from build123d import *

# Parameters (mm, degrees)
ESQUISSE1_W             = 160
ESQUISSE1_H             = 80
BOSS_EXTRU_1_DEPTH      = 2
ENL_V_MAT_EXTRU_2_DEPTH = 2
ENL_V_MAT_EXTRU_3_DEPTH = 2
ENL_V_MAT_EXTRU_4_REACH = 4
ESQUISSE8_W             = 8
ESQUISSE8_H             = 48


with BuildPart() as part:
    # Esquisse1 → Boss.-Extru.1 (new body)
    with BuildSketch(Plane(origin=(0, 0, 0), x_dir=(1, 0, 0), z_dir=(0, 1, 0))):
        with Locations((80, 40)):
            Rectangle(ESQUISSE1_W, ESQUISSE1_H)
    extrude(amount=BOSS_EXTRU_1_DEPTH)

    # Esquisse2 → Enlèv. mat.-Extru.2 (cut)
    with BuildSketch(Plane(origin=(0, 2, 0), x_dir=(1, 0, 0), z_dir=(0, 1, 0))):
        Polygon((0, 50), (30, 80), (0, 80), align=None)
        Polygon((130, 80), (160, 50), (160, 80), align=None)
        Polygon((130, 0), (160, 30), (160, 0), align=None)
        Polygon((0, 30), (30, 0), (0, 0), align=None)
    extrude(amount=-ENL_V_MAT_EXTRU_2_DEPTH, mode=Mode.SUBTRACT)

    # Esquisse7 → Enlèv. mat.-Extru.3 (cut)
    with BuildSketch(Plane(origin=(0, 2, 0), x_dir=(1, 0, 0), z_dir=(0, 1, 0))):
        with BuildLine():
            Line((62.95, 23), (62.95, 33))
            ThreePointArc((62.95, 33), (64, 34.05), (65.05, 33))
            Line((65.05, 33), (65.05, 23))
            ThreePointArc((65.05, 23), (64, 21.95), (62.95, 23))
        make_face()
        with BuildLine():
            Line((50.95, 23), (50.95, 33))
            ThreePointArc((50.95, 33), (52, 34.05), (53.05, 33))
            Line((53.05, 33), (53.05, 23))
            ThreePointArc((53.05, 23), (52, 21.95), (50.95, 23))
        make_face()
        with BuildLine():
            Line((50.95, 47), (50.95, 57))
            ThreePointArc((50.95, 57), (52, 58.05), (53.05, 57))
            Line((53.05, 57), (53.05, 47))
            ThreePointArc((53.05, 47), (52, 45.95), (50.95, 47))
        make_face()
        with BuildLine():
            Line((62.95, 47), (62.95, 57))
            ThreePointArc((62.95, 57), (64, 58.05), (65.05, 57))
            Line((65.05, 57), (65.05, 47))
            ThreePointArc((65.05, 47), (64, 45.95), (62.95, 47))
        make_face()
        with BuildLine():
            Line((97.05, 47), (97.05, 57))
            ThreePointArc((97.05, 57), (96, 58.05), (94.95, 57))
            Line((94.95, 57), (94.95, 47))
            ThreePointArc((94.95, 47), (96, 45.95), (97.05, 47))
        make_face()
        with BuildLine():
            Line((109.05, 47), (109.05, 57))
            ThreePointArc((109.05, 57), (108, 58.05), (106.95, 57))
            Line((106.95, 57), (106.95, 47))
            ThreePointArc((106.95, 47), (108, 45.95), (109.05, 47))
        make_face()
        with BuildLine():
            Line((109.05, 23), (109.05, 33))
            ThreePointArc((109.05, 33), (108, 34.05), (106.95, 33))
            Line((106.95, 33), (106.95, 23))
            ThreePointArc((106.95, 23), (108, 21.95), (109.05, 23))
        make_face()
        with BuildLine():
            Line((97.05, 23), (97.05, 33))
            ThreePointArc((97.05, 33), (96, 34.05), (94.95, 33))
            Line((94.95, 33), (94.95, 23))
            ThreePointArc((94.95, 23), (96, 21.95), (97.05, 23))
        make_face()
    extrude(amount=-ENL_V_MAT_EXTRU_3_DEPTH, mode=Mode.SUBTRACT)

    # Esquisse8 → Enlèv. mat.-Extru.4 (cut, up to next)
    with BuildSketch(Plane(origin=(0, 2, 0), x_dir=(1, 0, 0), z_dir=(0, 1, 0)), mode=Mode.PRIVATE) as enl_v_mat_extru_4_sk1:
        with Locations((124.5, 40)):
            Rectangle(ESQUISSE8_W, ESQUISSE8_H)
    enl_v_mat_extru_4_tool1 = extrude(enl_v_mat_extru_4_sk1.sketch, amount=-ENL_V_MAT_EXTRU_4_REACH, mode=Mode.PRIVATE) & part.part
    add(enl_v_mat_extru_4_tool1.solids().sort_by_distance((124.5, 2, -40))[0], mode=Mode.SUBTRACT)
    # Esquisse8 → Enlèv. mat.-Extru.4 (cut, up to next)
    with BuildSketch(Plane(origin=(0, 2, 0), x_dir=(1, 0, 0), z_dir=(0, 1, 0)), mode=Mode.PRIVATE) as enl_v_mat_extru_4_sk2:
        with Locations((35.5, 40)):
            Rectangle(ESQUISSE8_W, ESQUISSE8_H)
    enl_v_mat_extru_4_tool2 = extrude(enl_v_mat_extru_4_sk2.sketch, amount=-ENL_V_MAT_EXTRU_4_REACH, mode=Mode.PRIVATE) & part.part
    add(enl_v_mat_extru_4_tool2.solids().sort_by_distance((35.5, 2, -40))[0], mode=Mode.SUBTRACT)


solid = part.part
Could you check a few things on this model? Use its own coordinates, in mm. Give positions to 0.01 mm unless a question says otherwise; leave off trailing zeros. Loops run counter-clockwise (first coordinate to the right, second up) from the corner with the lowest first, then second, coordinate; pieces in that order, holes last. Notation, with made-up numbers: (36.25, -38.75) -> (68.25, -38.75) arc R19 ccw to (68.25, -22.75) -> close; hole circle Ø6 at (11.25, 61). An arc over 180 degrees is marked (long way). Answer as CSV lines item,"result". Start each with the question number.
(1) If we section it at D-D on z = -17.5: Write out the boundary of the cut face in (x, y).
(2) If we section it at A-A on x = 36: Write out the boundary of the cut face in (y, z).
(3) I need wall thicknesses on probe 1 along X at (y, z) = (1.5, -39); probe 2 along Z at (x, y) = (96, 1.8); probe 3 along Z at (x, y) = (127, 0.5). Which ranges of each line are inside material? Lowest first, please.
(4) I'm going to push flat-ended pins straight in: pin 1 Ø0.6 at (y, z) = (1, -53.5) entering from -X; pin 2 Ø1 at (y, z) = (0.5, -26.5) entering from -X; pin 3 Ø0.6 at (y, z) = (1.5, -27.5) entering from +X. Where does each tip first touch, or does it pass through?
(5) If we section it at B-B on z = -39.5: Write out the boundary of the cut face in (x, y), then the cut area to 3 significant figures.
(6) If we section it at C-C on y = 0.55: Count the separate pieces of the cut face and the enclosed holes in it, then the cut area to 3 significant figures.
Computed:
1,outline,"(12.5, 0) -> (31.5, 0) -> (31.5, 2) -> (12.5, 2) -> close; (39.5, 0) -> (120.5, 0) -> (120.5, 2) -> (39.5, 2) -> close; (128.5, 0) -> (147.5, 0) -> (147.5, 2) -> (128.5, 2) -> close"
2,outline,"(0, -80) -> (2, -80) -> (2, -64) -> (0, -64) -> close; (0, -16) -> (2, -16) -> (2, 0) -> (0, 0) -> close"
3,probe 1,"x = 0 to 31.5, 39.5 to 120.5, 128.5 to 160"
3,probe 2,"z = -80 to -58.05, -45.95 to -34.05, -21.95 to 0"
3,probe 3,"z = -80 to -64, -16 to 0"
4,pin 1,"stops at x = 3.2"
4,pin 2,"stops at x = 3"
4,pin 3,"stops at x = 157.8"
5,outline,"(0, 0) -> (31.5, 0) -> (31.5, 2) -> (0, 2) -> close; (39.5, 0) -> (120.5, 0) -> (120.5, 2) -> (39.5, 2) -> close; (128.5, 0) -> (160, 0) -> (160, 2) -> (128.5, 2) -> close"
5,area,"288 mm2"
6,separate pieces,"1"
6,enclosed holes,"10"
6,area,"10,000 mm2"
